Autodesk Fusion 360 part; units mm, degrees
sketch "Sketch1" plane through (0, 0, 0) normal (0, 1, 0) x (1, 0, 0)
  line L0 (0, 0) -> (57, 0)
  line L1 (57, 0) -> (57, 62.3)
  line L2 (57, 62.3) -> (0, 62.3)
  line L3 (0, 62.3) -> (0, 0)
  dimension "d1" = 57
  dimension "d2" = 62.3
extrude "Extrude1" add sketch "Sketch1" along normal blind 16
fillet "Fillet1" radius 5 2 edges at (28.5, 16, 0) (28.5, 16, -62.3)
sketch "Sketch2" plane through (0, 16, 0) normal (0, 1, 0) x (-1, 0, 0)
  line L0 (-57, -57.3) -> (0, -57.3)
  line L1 (0, -57.3) -> (0, -5)
  line L2 (0, -5) -> (-57, -5)
  line L3 (-57, -5) -> (-57, -57.3)
  line L4 (-55.4, -6.6) -> (-1.6, -6.6)
  line L5 (-1.6, -6.6) -> (-1.6, -55.7)
  line L6 (-1.6, -55.7) -> (-55.4, -55.7)
  line L7 (-55.4, -55.7) -> (-55.4, -6.6)
  dimension "d7" = 1.6
  dimension "d8" = 1.6
  dimension "d9" = 1.6
  dimension "d10" = 1.6
sketch "Sketch3" plane through (0, 0, 0) normal (0, -1, 0) x (1, 0, 0)
  line L0 (0, 0) -> (0, -62.3)
  line L1 (0, -62.3) -> (57, -62.3)
  line L2 (57, -62.3) -> (57, 0)
  line L3 (57, 0) -> (0, 0)
  circle A0 centre (28, -53.7) radius 1.8
  circle A1 centre (28, -38.67) radius 1.8
  circle A2 centre (28, -23.64) radius 1.8
  circle A3 centre (28, -8.61) radius 1.8
  dimension "d11" = 3.6
  dimension "d12" = 28
  dimension "d13" = 8.6
  dimension "d16" = 0
  dimension "d17" = 15.03
  dimension "d18" = 8.61
extrude "Extrude2" cut sketch "Sketch3" against normal blind 45 contours A0 | A1 | A2 | A3
equation "d9 = d7"
equation "d10 = d9"
equation "d13 = 6.8 mm + ( ( 3.6 / 2 ) * 1 mm )"
equation "d17 = 11.43 mm + 3.6 mm"
Here's how the part is built. I have some questions about the finished solid (model axes, mm). Round coordinates to 2 decimals unless told otherwise and drop trailing zeros. Loops run counter-clockwise (first coordinate to the right, second up) from the corner with the lowest first, then second, coordinate; pieces in that order, holes last. Notation, with made-up numbers: (-24, -3.5) - (3, -3.5) arc R20 ccw to (3, 8.5) - close; hole circle Ø1 at (27, -1). An arc over 180 degrees is marked (long way). One line per question, with ' | ' between items. Start each with the question number.
Q1. Will these pins go through, and if not, where does the flat tip stop? pin 1 (2 mm diameter, centred on x = 28, z = -38.67, fed in from -Y); pin 2 (1.5 mm diameter, centred on x = 36, y = 13.5, fed in from -Z).
Q2. I want a section at B-B (x = 28). Write out the boundary of the cut face in (y, z).
Q3. We'd pull the mould along Z, two halves only. Please class faces 1 (the flat face through (0, 8, -32)), 2 (the flat face through (29, 5, -62.3)), 3 (the cylindrical face through (28.968, 7.888, -37.152)): +Z half, -Z half, draft (parallel to the pull), parting line (faces both ways), or undercut.
Q4. Please list where these lines run through material, in increasing order: line 1 (Z direction, x = 28, y = 8); line 2 (Z direction, x = 27.5, y = 1.5); line 3 (Z direction, x = 42.5, y = 14). Write a range as [from, to].
Q5. I want a section at A-A (z = -8.61). Write out the boundary of the cut face in (x, y), then the cut area to 3 significant figures.
Response values:
1) pin 1: passes through | pin 2: stops at z = -61.98
2) outline: (0, -62.3) - (11, -62.3) arc R5 ccw to (16, -57.3) - (16, -55.5) - (0, -55.5) - close; (0, -51.9) - (16, -51.9) - (16, -40.47) - (0, -40.47) - close; (0, -36.87) - (16, -36.87) - (16, -25.44) - (0, -25.44) - close; (0, -21.84) - (16, -21.84) - (16, -10.41) - (0, -10.41) - close; (0, -6.81) - (16, -6.81) - (16, -5) arc R5 ccw to (11, 0) - (0, 0) - close
3) face 1: draft | face 2: -Z half | face 3: undercut
4) line 1: z = [-62.3, -55.5], [-51.9, -40.47], [-36.87, -25.44], [-21.84, -10.41], [-6.81, 0] | line 2: z = [-62.3, -55.43], [-51.97, -40.4], [-36.94, -25.37], [-21.91, -10.34], [-6.88, 0] | line 3: z = [-61.3, -1]
5) outline: (0, 0) - (26.2, 0) - (26.2, 16) - (0, 16) - close; (29.8, 0) - (57, 0) - (57, 16) - (29.8, 16) - close | area: 854 mm²
